from build123d import *

# Parameters (mm, degrees)
SKETCH_1_R      = 2
SKETCH_3_R      = 3
EXTRUDE_1_DEPTH = 28.5
SKETCH_4_R      = 3
EXTRUDE_2_DEPTH = 28.5
FILLET_1_R      = 1.5


with BuildPart() as part:
    # 스윕1: sweep along a path in 스케치2
    with BuildLine(Plane(origin=(0, 0, 0), x_dir=(0, 0, -1), z_dir=(1, 0, 0))) as sweep_1_path:
        Line((0, 0), (0, 31.5))
        ThreePointArc((0, 31.5), (0.878679656, 33.621320344), (3, 34.5))
        Line((3, 34.5), (34.5, 34.5))
    # 스케치1 → 스윕1 (sweep)
    with BuildSketch(Plane(origin=(0, 0, 0), x_dir=(1, 0, 0), z_dir=(0, 1, 0))):
        Circle(SKETCH_1_R)
    sweep(path=sweep_1_path.line)

    # 스케치3 → 보스-돌출1 (add)
    with BuildSketch(Plane.XZ):
        with Locations(Location((0, 0, 0), (0, 0, 270))):
            Circle(SKETCH_3_R)
    extrude(amount=-EXTRUDE_1_DEPTH)

    # 스케치4 → 보스-돌출2 (add)
    with BuildSketch(Plane(origin=(0, 0, -34.5), x_dir=(-1, 0, 0), z_dir=(0, 0, -1))):
        with Locations((0, 34.5)):
            Circle(SKETCH_4_R)
    extrude(amount=-EXTRUDE_2_DEPTH)

    # 필렛1
    # the kernel refuses this fillet: 1.5 mm, written as the material it adds along each edge
    with BuildSketch(Plane(origin=(0, 28.5, 0), x_dir=(1, 0, 0), z_dir=(0, 0, 1))) as fillet_1_piece_1:
        with BuildLine():
            CenterArc((3.5, 1.414213562), FILLET_1_R, 180, 70.528779366)
            Line((2, 1.414213562), (1.97, 1.414213562))
            Line((1.97, 1.414213562), (1.97, 0))
            Line((1.97, 0), (2, -0.03))
            ThreePointArc((2, -0.03), (2.5, -0.03), (2.99, -0.028284271))
            Line((2.99, -0.028284271), (3, 0))
        make_face()
    revolve(axis=Axis((0, 28.5, 0), (0, 1, 0)))
    with BuildSketch(Plane(origin=(0, 34.5, -6), x_dir=(1, 0, 0), z_dir=(0, 1, 0))) as fillet_1_piece_2:
        with BuildLine():
            CenterArc((3.5, -1.414213562), FILLET_1_R, 109.471220634, 70.528779366)
            Line((3, 0), (2.99, 0.028284271))
            ThreePointArc((2.99, 0.028284271), (2.5, 0.03), (2, 0.03))
            Line((2, 0.03), (1.97, 0))
            Line((1.97, 0), (1.97, -1.414213562))
            Line((1.97, -1.414213562), (2, -1.414213562))
        make_face()
    revolve(axis=Axis((0, 34.5, -6), (0, 0, -1)))


solid = part.part
Geometry check sheet. Reference: the model listing, model coordinates, mm. A direction names the side the tool comes from. Round coordinates to 2 decimals unless told otherwise and drop trailing zeros. Write each loop counter-clockwise with the first axis right and the second up, starting at its lowest first coordinate (ties: lowest second). Pieces come first, ordered by that corner, then holes.
Item 1: Section check C-C (y = 15.5). Record the boundary of the cut face in (x, z), plus the area to 3 significant figures.
Determined:
outline: circle Ø6 at (0, 0)
area: 28.3 mm2
Item 2: Mould release check, pull along Y, two halves, no side actions. Record for faces 1 (the face through (0, 31, 2)), 2 (the face through (0.9, 14.05, -2.86)), 3 (the face through (0, 0, 0)), 4 (the face through (-0.434, 36.452, -3.804)): +Y half, -Y half, draft (parallel to the pull), parting line (faces both ways), or undercut.
Determined:
face 1: undercut
face 2: draft
face 3: -Y half
face 4: parting line
Item 3: Go/stop test with flat-tipped pins: pin 1 Ø2 at (x, z) = (0.5, -26) entering from -Y; pin 2 Ø3 at (x, y) = (-1, 24) entering from -Z. Record where each tip stops, or that it passes through.
Determined:
pin 1: stops at y = 31.5
pin 2: stops at z = -3
Item 4: Material ranges on line 1 along Y through (x, z) = (1.25, -9); line 2 along Y through (x, z) = (0, -22); line 3 along Z through (x, y) = (0, 30), recorded low to high.
Determined:
line 1: y = 31.77 to 37.23
line 2: y = 31.5 to 37.5
line 3: z = -2 to 2
Item 5: Section check A-A (x = 0). Record the boundary of the cut face in (y, z), plus the area to 3 significant figures.
Determined:
outline: (0, -3) - (28.5, -3) arc R1.5 cw to (29.91, -2) - (31.5, -2) arc R1 cw to (32.5, -3) - (32.5, -4.59) arc R1.5 cw to (31.5, -6) - (31.5, -34.5) - (37.5, -34.5) - (37.5, -6) arc R1.5 cw to (36.5, -4.59) - (36.5, -3) arc R5 ccw to (31.5, 2) - (29.91, 2) arc R1.5 cw to (28.5, 3) - (0, 3) - close
area: 386 mm2
Item 6: Section check B-B (z = -22). Record the boundary of the cut face in (x, y), plus the area to 3 significant figures.
Determined:
outline: circle Ø6 at (0, 34.5)
area: 28.3 mm2
Item 7: Access from +Z, -Z, +X, -X, +Y, -Y to the whole of each face (thin tool, end or side, straight path). Record for faces 5 (the face through (0.391, 37.474, -20.45)), 6 (the face through (0, 35, -34.5)).
Determined:
face 5: -Z
face 6: -Z, +X, -X, +Y, -Y
